Read the model definition and answer for the solid it produces. Units are mm, in the model's axes. A direction names the side the tool comes from. Coordinates: 2 decimals unless noted, no trailing zeros. Loops run counter-clockwise (first coordinate to the right, second up) from the corner with the lowest first, then second, coordinate; pieces in that order, holes last.
from build123d import *

# Parameters (mm, degrees)
BOSS_EXTRUDE1_DEPTH = 6.35
BOSS_EXTRUDE3_START = -0.288785
BOSS_EXTRUDE3_DEPTH = 3.798785
FILLET2_R           = 3.5


with BuildPart() as part:
    # Sketch2 → Boss-Extrude1 (new body, symmetric)
    with BuildSketch(Plane.XY):
        with BuildLine():
            Line((-34.874721139, 19.043380924), (-34.692361524, 18.805168895))
            ThreePointArc((-34.692361524, 18.805168895), (-37.96654895, 13.954446928), (-37.652863155, 8.110526316))
            ThreePointArc((-37.652863155, 8.110526316), (-32.263995686, 2.861184613), (-24.759487179, 3.388283261))
            ThreePointArc((-24.759487179, 3.388283261), (-19.9, 4.606687347), (-15.040512821, 3.388283261))
            ThreePointArc((-15.040512821, 3.388283261), (-7.536004314, 2.861184613), (-2.147136845, 8.110526316))
            ThreePointArc((-2.147136845, 8.110526316), (0, 9.569218559), (2.147136845, 8.110526316))
            ThreePointArc((2.147136845, 8.110526316), (7.536004314, 2.861184613), (15.040512821, 3.388283261))
            ThreePointArc((15.040512821, 3.388283261), (19.9, 4.606687347), (24.759487179, 3.388283261))
            ThreePointArc((24.759487179, 3.388283261), (33.900299187, 3.651616235), (38.298445746, 11.669103077))
            Line((38.298445746, 11.669103077), (38.298445746, 18.669103077))
            Line((38.298445746, 18.669103077), (38.598395064, 18.669103077))
            Line((38.598395064, 18.669103077), (38.598395064, 11.674617307))
            ThreePointArc((38.598395064, 11.674617307), (34.056830682, 3.395690678), (24.617948718, 3.123770759))
            ThreePointArc((24.617948718, 3.123770759), (19.9, 4.306687347), (15.182051282, 3.123770759))
            ThreePointArc((15.182051282, 3.123770759), (7.432830541, 2.579484111), (1.868239134, 8))
            ThreePointArc((1.868239134, 8), (0, 9.269218559), (-1.868239134, 8))
            ThreePointArc((-1.868239134, 8), (-7.432830541, 2.579484111), (-15.182051282, 3.123770759))
            ThreePointArc((-15.182051282, 3.123770759), (-19.9, 4.306687347), (-24.617948718, 3.123770759))
            ThreePointArc((-24.617948718, 3.123770759), (-32.367169459, 2.579484111), (-37.931760866, 8))
            ThreePointArc((-37.931760866, 8), (-38.255675546, 14.034483241), (-34.874721139, 19.043380924))
        make_face()
    extrude(amount=BOSS_EXTRUDE1_DEPTH, both=True)

    # Sketch6 → Boss-Extrude3 (add)
    with BuildSketch(Plane(origin=(38.598395064, 16.11055993, 0), x_dir=(0, 0, -1), z_dir=(1, 0, 0)).offset(BOSS_EXTRUDE3_START)):
        with BuildLine():
            Line((-1.5, 2.058543147), (1.5, 2.058543147))
            ThreePointArc((1.5, 2.058543147), (6, -2.441456853), (1.5, -6.941456853))
            Line((1.5, -6.941456853), (-1.5, -6.941456853))
            ThreePointArc((-1.5, -6.941456853), (-6, -2.441456853), (-1.5, 2.058543147))
        make_face()
    extrude(amount=BOSS_EXTRUDE3_DEPTH)

    # Fillet2
    fillet2_edges = [part.edges().sort_by_distance(p)[0] for p in [
        (42.108395064, 13.669103077, 6),
        (42.108395064, 9.169103077, 0),
        (42.108395064, 13.669103077, -6),
        (42.108395064, 18.169103077, 0),
    ]]
    fillet(fillet2_edges, radius=FILLET2_R)


solid = part.part
Item 1: Which of the six approach directions +Z, -Z, +X, -X, +Y, -Y give full straight-line access (tool end or side, diameter ignored) to faces 1 (the face through (-36.977, 6.189, -0.089)), 2 (the face through (38.298, 15, 0))?
Numbers:
face 1: +Z, -Z
face 2: +Z, -Z, +Y
Item 2: A cutting plane is placed at A-A on x = 35.5. Determine the outline of the cut face in (y, z), then the cut area to 3 significant figures.
Numbers:
outline: (4.48, -6.35) - (4.89, -6.35) - (4.89, 6.35) - (4.48, 6.35) - close
area: 5.23 mm2
Item 3: A cutting plane is placed at B-B on x = -17. Determine the outline of the cut face in (y, z).
Numbers:
outline: (3.88, -6.35) - (4.19, -6.35) - (4.19, 6.35) - (3.88, 6.35) - close
Item 4: Find the intervals of material crossed by line 1 along X through (y, z) = (6, 5.25); line 2 along X through (y, z) = (5.5, -0.75); line 3 along Y through (x, z) = (-20, 4.75), in increasing order.
Numbers:
line 1: x = -36.85 to -36.47, -3.33 to -2.95, 2.95 to 3.33, 36.47 to 36.85
line 2: x = -36.47 to -36.07, -3.73 to -3.33, 3.33 to 3.73, 36.07 to 36.47
line 3: y = 4.31 to 4.61
Item 5: Determine the mould class of faces 3 (the face through (41.11, 10.22, 0.02)), 4 (the face through (-0.04, 9.57, -0.09)) for opening direction X: released by +X, released by -X, zero draft, split by the parting line, or undercut.
Numbers:
face 3: released by +X
face 4: undercut
Item 6: Given pin 1 (4 mm diameter, centred on y = 6, z = -0.5, fed in from +X); pin 2 (3 mm diameter, centred on x = -22, z = -3.5, fed in from -Y); pin 3 (4 mm diameter, centred on y = 7.5, z = -1, fed in from -X), each flat-ended and moving along its own axis, determine where each tip first touches the part or whether it passes through.
Numbers:
pin 1: stops at x = 37.93
pin 2: stops at y = 3.64
pin 3: stops at x = -38.39
